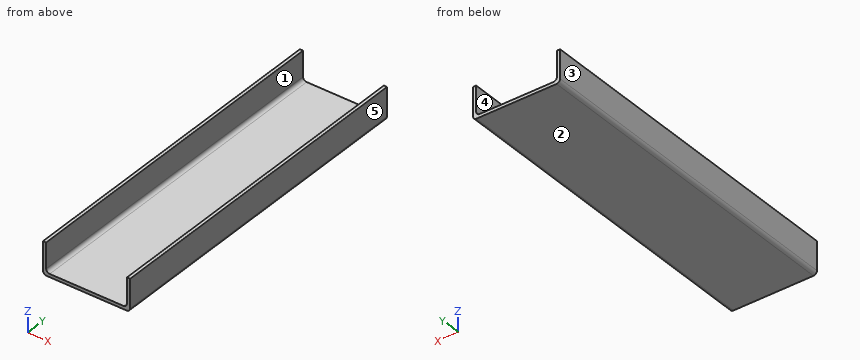
from build123d import *

# Parameters (mm, degrees)
F1_DEPTH = 480.5


with BuildPart() as f1:
    # F0 (on Front) → F1 (new body)
    with BuildSketch(Plane.XZ):
        with BuildLine():
            ThreePointArc((0, 5), (1.464466, 1.464466), (5, 0))
            Line((5, 0), (119, 0))
            ThreePointArc((119, 0), (122.535534, 1.464466), (124, 5))
            Line((124, 5), (124, 45.75))
            Line((124, 45.75), (119.5, 45.75))
            Line((119.5, 45.75), (119.5, 9.5))
            ThreePointArc((119.5, 9.5), (118.035534, 5.964466), (114.5, 4.5))
            Line((114.5, 4.5), (9.5, 4.5))
            ThreePointArc((9.5, 4.5), (5.964466, 5.964466), (4.5, 9.5))
            Line((4.5, 9.5), (4.5, 45.75))
            Line((4.5, 45.75), (0, 45.75))
            Line((0, 45.75), (0, 5))
        make_face()
    extrude(amount=F1_DEPTH)


solid = f1.part
The model under review builds one solid part; all positions refer to its coordinate system, in mm. Face numbers are marked on the shaded views. A direction names the side the tool comes from. Round coordinates to 2 decimals unless told otherwise and drop trailing zeros. Order: outer loops, then holes, each group sorted by start corner. A loop starts at its lowest first (then second) coordinate and runs counter-clockwise, first axis right, second up. Notation, with made-up numbers: (61, -33) -> (94, -33) arc R27 ccw to (94, 5) -> close; hole circle Ø10 at (32, 46). An arc over 180 degrees is marked (long way). Return JSON: item names as keys, results as strings.
1. Insertion check: P1, Ø3, axis at x = 79, y = -285.5, coming from the +Z side. The pin has a flat end and moves straight along its axis. Give the tip position at first contact, or say it passes through.
Answer block:
{"P1": "stops at z = 4.5"}
2. Take a section at C-C (x = 43.5). Write out the cut boundary in (y, z), then the cut area to 3 significant figures.
Answer block:
{"outline": "(-480.5, 0) -> (0, 0) -> (0, 4.5) -> (-480.5, 4.5) -> close", "area": "2,160 mm²"}
3. For the marked faces 4 and 5, list the 3-axis set-ups (+Z, -Z, +X, -X, +Y, -Y) from which the entire face can be reached by the end or side of a thin tool; tool diameter is ignored.
Answer block:
{"face 4": "+Z, +Y, -Y", "face 5": "+Z, -Z, +X, +Y, -Y"}
4. For L1, parallel to X at y = -330.5, z = 38; L2, parallel to Z at x = 25, y = -152.5; L3, parallel to X at y = -55.5, z = 6, list the stretches that pass through material, from the lowest coordinate up. Write a range as [from, to].
Answer block:
{"L1": "x = [0, 4.5], [119.5, 124]", "L2": "z = [0, 4.5]", "L3": "x = [0, 5.93], [118.07, 124]"}
5. Take a section at B-B (z = 40). Write out the cut boundary in (x, y), then the cut area to 3 significant figures.
Answer block:
{"outline": "(0, -480.5) -> (4.5, -480.5) -> (4.5, 0) -> (0, 0) -> close; (119.5, -480.5) -> (124, -480.5) -> (124, 0) -> (119.5, 0) -> close", "area": "4,320 mm²"}
6. Take a section at A-A (y = -314.5). Write out the cut boundary in (x, z).
Answer block:
{"outline": "(0, 5) arc R5 ccw to (5, 0) -> (119, 0) arc R5 ccw to (124, 5) -> (124, 45.75) -> (119.5, 45.75) -> (119.5, 9.5) arc R5 cw to (114.5, 4.5) -> (9.5, 4.5) arc R5 cw to (4.5, 9.5) -> (4.5, 45.75) -> (0, 45.75) -> close"}
7. The part is to be moulded in two halves that separate along X. For the marked faces 1, 2 and 3, say which applies: +X half, -X half, draft (parallel to the pull), parting line (faces both ways), or undercut.
Answer block:
{"face 1": "undercut", "face 2": "draft", "face 3": "-X half"}
